Source: three-view drawing plus pictorial views. Frame: mm from the lowest corner of the part. Give positions to 0.01 mm unless a question says otherwise; leave off trailing zeros. Loops run counter-clockwise (first coordinate to the right, second up) from the corner with the lowest first, then second, coordinate; pieces in that order, holes last. Notation, with made-up numbers: (18, 16.5) - (64, 16.5) arc R19 cw to (64, 31.5) - close; hole circle Ø9 at (4.25, -35). An arc over 180 degrees is marked (long way). Answer as a JSON object with one key per item and string values. Group by question number.
(1) Section query B-B (x = 16). Return loops of the section in (y, z) (1 decimal).
(2) Section query A-A (z = 63.5). Return loops of the section in (x, y).
(3) Section query D-D (y = 1.5). Return loops of the section in (x, z).
(4) Material intervals for L1, parallel to Z at x = 19.5, y = 0.55 (1 decimal); L2, parallel to Z at x = 21, y = 1.85; L3, parallel to X at y = 2.1, z = 62 (1 decimal), sorted ascending.
(5) Section query C-C (x = 58.5). Return loops of the section in (y, z).
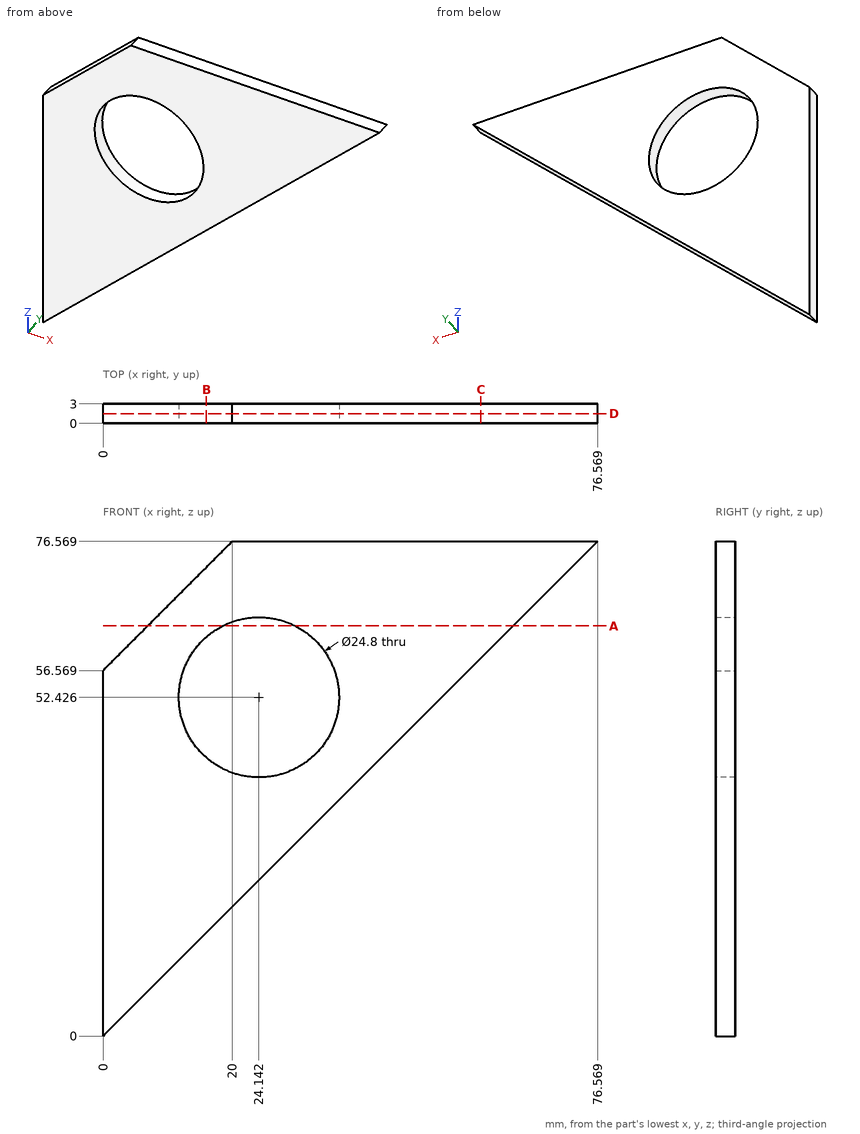
Recorded:
{
 "1": {"outline": "(0, 16) - (3, 16) - (3, 43.1) - (0, 43.1) - close; (0, 61.8) - (3, 61.8) - (3, 72.6) - (0, 72.6) - close"},
 "2": {"outline": "(6.93, 0) - (18.56, 0) - (18.56, 3) - (6.93, 3) - close; (29.72, 0) - (63.5, 0) - (63.5, 3) - (29.72, 3) - close"},
 "3": {"outline": "(0, 0) - (76.57, 76.57) - (20, 76.57) - (0, 56.57) - close; hole circle Ø24.8 at (24.14, 52.43)"},
 "4": {"L1": "z = 19.5 to 40.9, 63.9 to 76.1", "L2": "z = 21 to 40.43, 64.42 to 76.57", "L3": "x = 5.4 to 16.3, 32 to 62"},
 "5": {"outline": "(0, 58.5) - (3, 58.5) - (3, 76.57) - (0, 76.57) - close"}
}
